Check sheet for the drawn part. Datum: minimum x, y, z corner. Units: mm. Round coordinates to 2 decimals unless told otherwise and drop trailing zeros. Write each loop counter-clockwise with the first axis right and the second up, starting at its lowest first coordinate (ties: lowest second). Pieces come first, ordered by that corner, then holes. Notation, with made-up numbers: (83, -0.5) - (139, -0.5) arc R29 ccw to (139, 26.5) - close; hole circle Ø9 at (71.25, -7). An arc over 180 degrees is marked (long way). Return JSON: item names as keys, results as strings. Group by question number.
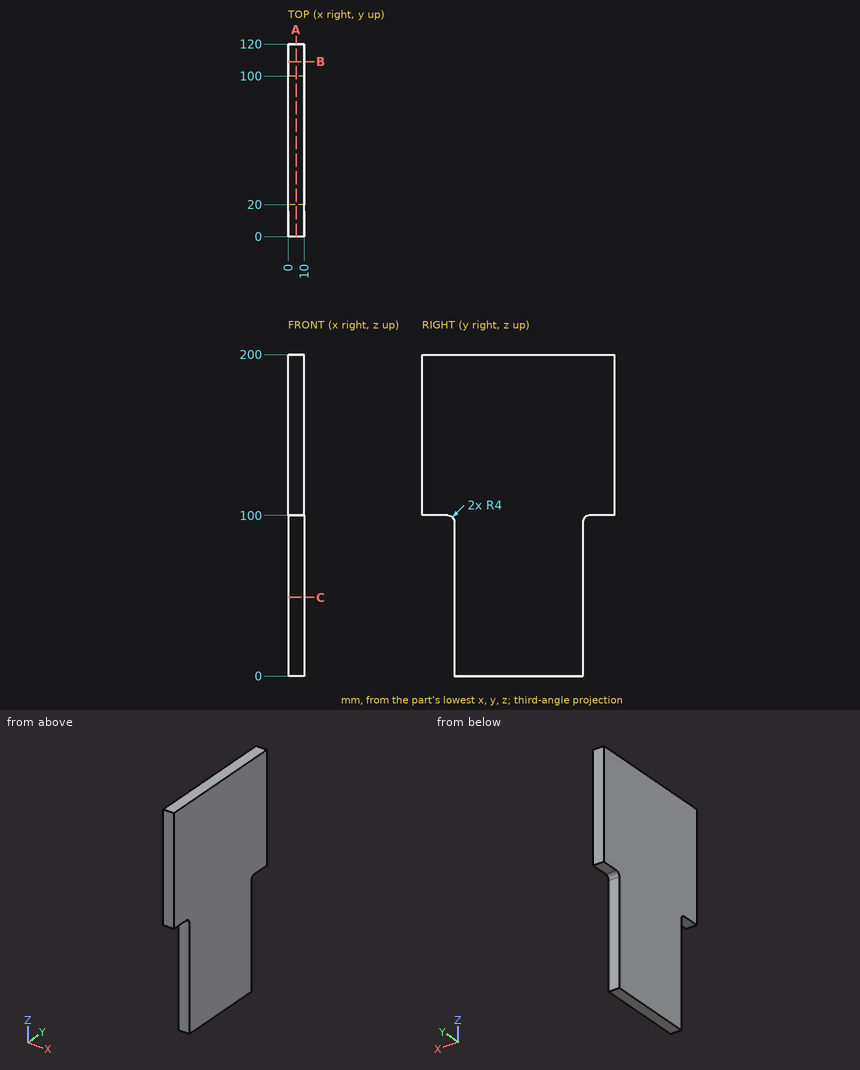
1. Section check B-B (y = 109). Enter the section's corners in (x, z).
2. Section check C-C (z = 49). Enter the section's corners in (x, y).
3. Material ranges on line 1 along Y through (x, z) = (7, 33); line 2 along Z through (x, y) = (1.75, 9); line 3 along Y through (x, z) = (1.5, 98.5), recorded low to high.
4. Depth check by flat-ended pin: pin 1 Ø5 at (x, z) = (3.5, 32) entering from +Y; pin 2 Ø3 at (x, z) = (4, 43.5) entering from -Y; pin 3 Ø5 at (x, y) = (4, 6) entering from -Z. Enter the tip coordinate at first touch or a pass-through.
5. Section check A-A (x = 5). Enter the section's corners in (y, z).
Result sheet:
{
 "1": {"outline": "(0, 100) - (10, 100) - (10, 200) - (0, 200) - close"},
 "2": {"outline": "(0, 20) - (10, 20) - (10, 100) - (0, 100) - close"},
 "3": {"line 1": "y = 20 to 100", "line 2": "z = 100 to 200", "line 3": "y = 19.12 to 100.88"},
 "4": {"pin 1": "stops at y = 100", "pin 2": "stops at y = 20", "pin 3": "stops at z = 100"},
 "5": {"outline": "(0, 100) - (16, 100) arc R4 cw to (20, 96) - (20, 0) - (100, 0) - (100, 96) arc R4 cw to (104, 100) - (120, 100) - (120, 200) - (0, 200) - close"}
}
